Here's how the part is built. I have some questions about the finished solid (model axes, mm). A direction names the side the tool comes from. Give positions to 0.01 mm unless a question says otherwise; leave off trailing zeros. Order: outer loops, then holes, each group sorted by start corner. A loop starts at its lowest first (then second) coordinate and runs counter-clockwise, first axis right, second up. Notation, with made-up numbers: (-23.5, 84.25) - (-6.5, 84.25) arc R19 cw to (-6.5, 116.25) - close; hole circle Ø7 at (33, 63.5). An arc over 180 degrees is marked (long way). One line per question, with ' | ' between items.
from build123d import *

# Parameters (mm, degrees)
SKETCH1_W           = 120
SKETCH1_H           = 120
BOSS_EXTRUDE1_DEPTH = 90
FILLET1_R           = 10
CUT_EXTRUDE4_DEPTH  = 20
SHELL1_T            = -4


with BuildPart() as part:
    # Sketch1 → Boss-Extrude1 (new body)
    with BuildSketch(Plane.XY):
        Rectangle(SKETCH1_W, SKETCH1_H)
    extrude(amount=BOSS_EXTRUDE1_DEPTH)

    # Fillet1
    fillet1_edges = [part.edges().sort_by_distance(p)[0] for p in [
        (60, -60, 45),
        (-60, -60, 45),
        (-60, 60, 45),
        (60, 60, 45),
    ]]
    fillet(fillet1_edges, radius=FILLET1_R)

    # Sketch4 → Cut-Extrude4 (cut)
    with BuildSketch(Plane.XY.offset(90)):
        with BuildLine():
            Line((-60, 50), (-60, -50))
            ThreePointArc((-60, -50), (-57.071067812, -57.071067812), (-50, -60))
            Line((-50, -60), (50, -60))
            ThreePointArc((50, -60), (57.071067812, -57.071067812), (60, -50))
            Line((60, -50), (60, 50))
            ThreePointArc((60, 50), (57.071067812, 57.071067812), (50, 60))
            Line((50, 60), (-50, 60))
            ThreePointArc((-50, 60), (-57.071067812, 57.071067812), (-60, 50))
        make_face()
        with BuildLine():
            Line((-58, 50), (-58, -50))
            ThreePointArc((-58, -50), (-55.656854249, -55.656854249), (-50, -58))
            Line((-50, -58), (50, -58))
            ThreePointArc((50, -58), (55.656854249, -55.656854249), (58, -50))
            Line((58, -50), (58, 50))
            ThreePointArc((58, 50), (55.656854249, 55.656854249), (50, 58))
            Line((50, 58), (-50, 58))
            ThreePointArc((-50, 58), (-55.656854249, 55.656854249), (-58, 50))
        make_face(mode=Mode.SUBTRACT)
    extrude(amount=-CUT_EXTRUDE4_DEPTH, mode=Mode.SUBTRACT)

    # Shell1
    shell1_openings = [part.faces().sort_by_distance(p)[0] for p in [
        (0, 0, 90),
    ]]
    offset(amount=SHELL1_T, openings=shell1_openings, kind=Kind.INTERSECTION)


solid = part.part
1) Thinking about a two-plate mould opening in Y: for faces 4 (the face through (-1, 1, 4)), 5 (the face through (55.719, 55.594, 80.14)), 6 (the face through (-55.719, -55.594, 80.14)), which applies, +Y half, -Y half, draft (parallel to the pull), parting line (faces both ways), or undercut?
Model answer:
face 4: undercut | face 5: +Y half | face 6: -Y half
2) On a 3-axis mill with a long thin cutter (end or side, diameter ignored), from which of +Z, -Z, +X, -X, +Y, -Y can I reach the whole of each face in a straight line? I mean faces 1 (the face through (-55.594, 55.719, 80.14)), 2 (the face through (-1, 56, 35)), 3 (the face through (58, -1, 80)). Say none if no direction works.
Model answer:
face 1: +Z, -X, +Y | face 2: none | face 3: +Z, +X, +Y, -Y
3) I want a section at A-A (z = 64). List the corners of the cut face in (x, y) for me, plus the area to 3 significant figures.
Model answer:
outline: (-60, -50) arc R10 ccw to (-50, -60) - (50, -60) arc R10 ccw to (60, -50) - (60, 50) arc R10 ccw to (50, 60) - (-50, 60) arc R10 ccw to (-60, 50) - close; hole (-56, -50) arc R6 ccw to (-50, -56) - (50, -56) arc R6 ccw to (56, -50) - (56, 50) arc R6 ccw to (50, 56) - (-50, 56) arc R6 ccw to (-56, 50) - close | area: 1,800 mm2
4) I want a section at B-B (y = 3.5). List the corners of the cut face in (x, z) for me.
Model answer:
outline: (-60, 0) - (60, 0) - (60, 70) - (58, 70) - (58, 90) - (54, 90) - (54, 66) - (56, 66) - (56, 4) - (-56, 4) - (-56, 66) - (-54, 66) - (-54, 90) - (-58, 90) - (-58, 70) - (-60, 70) - close
5) I'm going to push flat-ended pins straight in: P1, Ø1, axis at x = -38, y = -26.5, coming from the +Z side; P2, Ø1, axis at y = -38, z = 72.5, coming from the -X side; P3, Ø19, axis at y = -8.5, z = 73.5, coming from the -X side; P4, Ø3, axis at x = -41, z = 73.5, coming from the +Y side. Where does each tip first touch, or does it pass through?
Model answer:
P1: stops at z = 4 | P2: stops at x = -58 | P3: stops at x = -60 | P4: stops at y = 58
6) I want a section at D-D (z = 74.5). List the corners of the cut face in (x, y) for me, plus the area to 3 significant figures.
Model answer:
outline: (-58, -50) arc R8 ccw to (-50, -58) - (50, -58) arc R8 ccw to (58, -50) - (58, 50) arc R8 ccw to (50, 58) - (-50, 58) arc R8 ccw to (-58, 50) - close; hole (-54, -50) arc R4 ccw to (-50, -54) - (50, -54) arc R4 ccw to (54, -50) - (54, 50) arc R4 ccw to (50, 54) - (-50, 54) arc R4 ccw to (-54, 50) - close | area: 1,750 mm2
7) Please list where these lines run through material, in increasing order: L1, parallel to X at y = -15, z = 46; L2, parallel to Y at x = -7.5, z = 75.
Model answer:
L1: x = -60 to -56, 56 to 60 | L2: y = -58 to -54, 54 to 58
